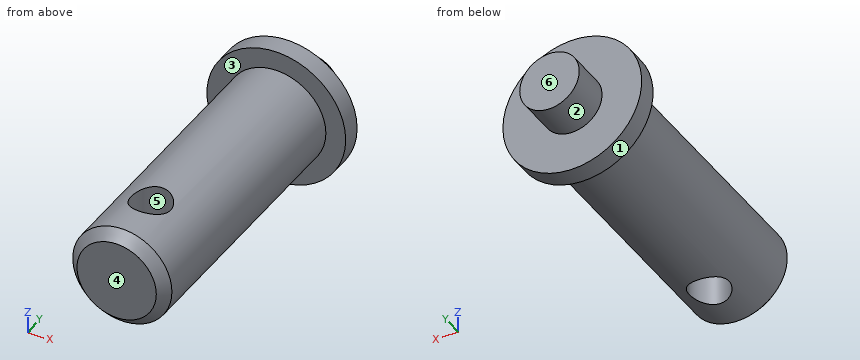
Autodesk Inventor part; units mm, degrees
ref_plane "YZ Plane" through (0, 0, 0) normal (1, 0, 0) x (0, 1, 0)
ref_plane "XZ Plane" through (0, 0, 0) normal (0, 1, 0) x (-1, 0, 0)
ref_plane "XY Plane" through (0, 0, 0) normal (0, 0, 1) x (1, 0, 0)
sketch "Sketch1" plane through (0, 0, 0) normal (0, 0, 1) x (1, 0, 0)
  line L0 (0, 8.5) -> (0, -8.5)
  line L1 (0, -8.5) -> (2.5, -8.5)
  line L2 (2.5, -8.5) -> (2.5, 5.5)
  line L3 (2.5, 5.5) -> (3.5, 5.5)
  line L4 (3.5, 5.5) -> (3.5, 6.5)
  line L5 (3.5, 6.5) -> (1.5, 6.5)
  line L6 (1.5, 6.5) -> (1.5, 8.5)
  line L7 (1.5, 8.5) -> (0, 8.5)
  point P0 (0, 0)
  point P1 (0, 0)
  dimension "d0" = 3
  dimension "d1" = 5
  dimension "d2" = 7
  dimension "d3" = 2
  dimension "d4" = 1
  dimension "d5" = 17
revolve "Revolution1" add sketch "Sketch1" angle 360 about axis through (0, 8.5, 0) along (0, -1, 0)
sketch "Sketch2" plane through (0, 0, 0) normal (0, 0, 1) x (1, 0, 0)
  circle A0 centre (0, -5.5) radius 1
  line L0 (-2.5, -8.5) -> (2.5, -8.5)
  point P0 (0, 0)
  point P1 (0, -8.5)
  dimension "d7" = 2
  dimension "d8" = 4
extrude "Extrusion1" cut sketch "Sketch2" along normal through all both and the other way through all
chamfer "Chamfer1" distance 0.5 angle 45 1 edges at (-2.5, -8.5, 0)
properties part number "Locking Pin"
Geometry: final body of the model. Coordinates: model frame, mm. Face numbers are marked on the shaded views. A direction names the side the tool comes from. Give positions to 0.01 mm unless a question says otherwise; leave off trailing zeros. Loops run counter-clockwise (first coordinate to the right, second up) from the corner with the lowest first, then second, coordinate; pieces in that order, holes last. Notation, with made-up numbers: (50.5, 54.25) - (77.5, 54.25) arc R17 cw to (77.5, 61.25) - close; hole circle Ø5 at (-20.75, 68). An arc over 180 degrees is marked (long way). Answer as CSV lines item,"result". Start each with the question number.
(1) Pin query (flat end, axial travel): P1, Ø1, axis at x = 1.5, y = 0, coming from the -Z side; P2, Ø2, axis at x = 2, y = 5, coming from the -Z side; P3, Ø1.5, axis at x = -2.5, z = 1.5, coming from the -Y side. Return the tip coordinate at first contact, or that it passes through.
(2) Section query D-D (y = 2.25). Output: boundary loops of the cut face in (x, z), and give its area (3 significant figures).
(3) Mould query, pull axis Y, two halves, no side actions, for the marked faces 4, 5 and 6. Classes: +Y half, -Y half, draft (parallel to the pull), parting line (faces both ways), or undercut.
(4) Section query C-C (y = -5.5). Output: boundary loops of the cut face in (x, z), and give its area (3 significant figures).
(5) Ray query, line 1 along Y through (x, z) = (0, -1.45); line 2 along X through (y, z) = (-5.5, -0.05); line 3 along X through (y, z) = (-5.5, 0.8). Return the intervals inside material, ascending. Write a range as [from, to].
(6) Reachability of the marked faces 1, 2 and 3 from +Z, -Z, +X, -X, +Y, -Y: full face, straight path, thin tool, end or side. Return the list, or none.
(7) Section query A-A (x = 0). Output: boundary loops of the cut face in (y, z).
(8) Section query B-B (z = 0). Output: boundary loops of the cut face in (x, y).
Worked answers:
1,P1,"stops at z = -2.29"
1,P2,"stops at z = -3.31"
1,P3,"stops at y = -8.33"
2,outline,"circle Ø5 at (0, 0)"
2,area,"19.6 mm^2"
3,face 4,"-Y half"
3,face 5,"undercut"
3,face 6,"+Y half"
4,outline,"(-1, -2.29) - (-1, 2.29) arc R2.5 ccw to start; (1, -2.29) arc R2.5 ccw to (1, 2.29) - close"
4,area,"9.91 mm^2"
5,line 1,"y = [-8.5, -6.5], [-4.5, 8.5]"
5,line 2,"x = [-2.5, -1], [1, 2.5]"
5,line 3,"x = [-2.37, -1], [1, 2.37]"
6,face 1,"+Y, -Y"
6,face 2,"+Y"
6,face 3,"-Y"
7,outline,"(-8.5, -2) - (-8, -2.5) - (-6.5, -2.5) - (-6.5, 2.5) - (-8, 2.5) - (-8.5, 2) - close; (-4.5, -2.5) - (5.5, -2.5) - (5.5, -3.5) - (6.5, -3.5) - (6.5, -1.5) - (8.5, -1.5) - (8.5, 1.5) - (6.5, 1.5) - (6.5, 3.5) - (5.5, 3.5) - (5.5, 2.5) - (-4.5, 2.5) - close"
8,outline,"(-3.5, 5.5) - (-2.5, 5.5) - (-2.5, -8) - (-2, -8.5) - (2, -8.5) - (2.5, -8) - (2.5, 5.5) - (3.5, 5.5) - (3.5, 6.5) - (1.5, 6.5) - (1.5, 8.5) - (-1.5, 8.5) - (-1.5, 6.5) - (-3.5, 6.5) - close; hole circle Ø2 at (0, -5.5)"
